Here's how the part is built. I have some questions about the finished solid (model axes, mm). A direction names the side the tool comes from. Coordinates: 2 decimals unless noted, no trailing zeros. Write each loop counter-clockwise with the first axis right and the second up, starting at its lowest first coordinate (ties: lowest second). Pieces come first, ordered by that corner, then holes. Notation, with made-up numbers: (-14.5, 4) -> (43.5, 4) arc R6 cw to (43.5, 13) -> close; hole circle Ø6 at (67, 9). An arc over 180 degrees is marked (long way). Use a Markdown table: item, result. Add a question column.
Item 1: Imagine slicing it at D-D, the plane x = 14. Write out the boundary of the cut face in (y, z).
Item 2: Will these pins go through, and if not, where does the flat tip stop? pin 1 Ø1.1 at (x, y) = (30, 19) entering from +Z; pin 2 Ø2.5 at (x, z) = (-2.125, -7) entering from -Y; pin 3 Ø0.7 at (x, y) = (-4, 18.5) entering from +Z.
Item 3: Imagine slicing it at A-A, the plane x = 4.5. Write out the boundary of the cut face in (y, z), and give its area (3 significant figures).
Item 4: If I drill on line 1 along X through (y, z) = (18.6, -7) (3 decimals); line 2 along Y through (x, z) = (19.5, -4.5); line 3 along X through (y, z) = (20.5, -1), over which ranges is the centre line in solid material (lowest first)? Write a range as from..to.
Item 5: Imagine slicing it at B-B, the plane z = -5. Write out the boundary of the cut face in (x, y).
Item 6: If we mould it in two halves opening along Z, with no side actions, what happens to faces 5 (the cylindrical face through (20.666, 28.723, -8.817)), 6 (the flat face through (-0.7, 19.2, -7.1)), 7 (the cylindrical face through (-1.126, 18.46, -6.965)), 8 (the flat face through (13, 12, 0))? For each: pulls with the +Z half, pulls with the -Z half, needs draft (parallel to the pull), parting line crosses it, or undercut.
Item 7: Imagine slicing it at C-C, the plane y = 7.5. Write out the boundary of the cut face in (x, z), and give its area (3 significant figures).
Item 8: On a 3-axis mill with a long thin cutter (end or side, diameter ignored), from which of +Z, -Z, +X, -X, +Y, -Y can I reach the whole of each face in a straight line? I mean faces 1 (the flat face through (26, 21, -7)), 2 (the flat face through (-0.7, 17.7, -7.1)), 3 (the flat face through (26.7, 17.7, -7.1)), 4 (the flat face through (16, 26.8, -7)). Say none if no direction works.
```python
from build123d import *

# Parameters (mm, degrees)
SKETCH1_W           = 26
SKETCH1_H           = 14
BOSS_EXTRUDE1_DEPTH = 22.7
SKETCH2_W           = 34.5
SKETCH2_H           = 14
BOSS_EXTRUDE2_DEPTH = 1.5
CHAMFER1_SIZE       = 1
SKETCH3_R           = 7
BOSS_EXTRUDE3_DEPTH = 26.8
SKETCH4_R           = 2.465
BOSS_EXTRUDE4_DEPTH = 3.9
SKETCH5_R           = 1
CUT_EXTRUDE1_DEPTH  = 39.466901357
SKETCH7_W           = 4.817382001
SKETCH7_H           = 1.25
SKETCH7_W_2         = 10.544713936
CUT_EXTRUDE2_DEPTH  = 39.466901357


with BuildPart() as part:
    # Sketch1 → Boss-Extrude1 (new body)
    with BuildSketch(Plane(origin=(0, 0, 0), x_dir=(1, 0, 0), z_dir=(0, 1, 0))):
        with Locations((13, 7)):
            Rectangle(SKETCH1_W, SKETCH1_H)
    extrude(amount=BOSS_EXTRUDE1_DEPTH)

    # Sketch2 → Boss-Extrude2 (add)
    with BuildSketch(Plane(origin=(0, 19.2, 0), x_dir=(1, 0, 0), z_dir=(0, 1, 0))):
        with Locations((13, 7)):
            Rectangle(SKETCH2_W, SKETCH2_H)
    extrude(amount=-BOSS_EXTRUDE2_DEPTH)

    # Chamfer1
    chamfer1_edges = [part.edges().sort_by_distance(p)[0] for p in [
        (-4.25, 18.45, -14),
        (30.25, 18.45, 0),
        (-4.25, 18.45, 0),
        (30.25, 18.45, -14),
    ]]
    chamfer(chamfer1_edges, length=CHAMFER1_SIZE)

    # Sketch3 → Boss-Extrude3 (add)
    with BuildSketch(Plane.XZ):
        with Locations(Location((19, -7, 0), (0, 0, 270))):
            Circle(SKETCH3_R)
    extrude(amount=-BOSS_EXTRUDE3_DEPTH)

    # Sketch4 → Boss-Extrude4 (add)
    with BuildSketch(Plane(origin=(0, 26.8, 0), x_dir=(1, 0, 0), z_dir=(0, 1, 0))):
        with Locations(Location((19, 7, 0), (0, 0, 270))):
            Circle(SKETCH4_R)
    extrude(amount=BOSS_EXTRUDE4_DEPTH)

    # Sketch5 → Cut-Extrude1 (cut, through all)
    with BuildSketch(Plane(origin=(0, 19.2, 0), x_dir=(1, 0, 0), z_dir=(0, 1, 0))):
        with Locations(Location((28.125, 7, 0), (0, 0, 270))):
            Circle(SKETCH5_R)
        with Locations(Location((-2.125, 7, 0), (0, 0, 270))):
            Circle(SKETCH5_R)
    extrude(amount=-CUT_EXTRUDE1_DEPTH, mode=Mode.SUBTRACT)

    # Sketch7 → Cut-Extrude2 (cut, through all)
    with BuildSketch(Plane(origin=(0, 19.2, 0), x_dir=(1, 0, 0), z_dir=(0, 1, 0))):
        with Locations((30.431785983, 7)):
            Rectangle(SKETCH7_W, SKETCH7_H)
        with Locations((-7.29545195, 7)):
            Rectangle(SKETCH7_W_2, SKETCH7_H)
    extrude(amount=-CUT_EXTRUDE2_DEPTH, mode=Mode.SUBTRACT)


solid = part.part
```
Ans:
| question | item | result |
|---|---|---|
| 1 | outline | (0, -14) -> (22.7, -14) -> (22.7, -11.9) -> (26.8, -11.9) -> (26.8, -2.1) -> (22.7, -2.1) -> (22.7, 0) -> (0, 0) -> close |
| 2 | pin 1 | stops at z = -0.2 |
| 2 | pin 2 | stops at y = 17.7 |
| 2 | pin 3 | stops at z = -0.4 |
| 3 | outline | (0, -14) -> (22.7, -14) -> (22.7, 0) -> (0, 0) -> close |
| 3 | area | 318 mm^2 |
| 4 | line 1 | x = -1.125..27.125 |
| 4 | line 2 | y = 0..26.8 |
| 4 | line 3 | x = 0..26 |
| 5 | outline | (-4.25, 17.7) -> (0, 17.7) -> (0, 0) -> (26, 0) -> (26, 17.7) -> (30.25, 17.7) -> (30.25, 19.2) -> (26, 19.2) -> (26, 22.7) -> (25.71, 22.7) -> (25.71, 26.8) -> (20.44, 26.8) -> (20.44, 30.7) -> (17.56, 30.7) -> (17.56, 26.8) -> (12.29, 26.8) -> (12.29, 22.7) -> (0, 22.7) -> (0, 19.2) -> (-4.25, 19.2) -> close |
| 6 | face 5 | parting line crosses it |
| 6 | face 6 | needs draft |
| 6 | face 7 | undercut |
| 6 | face 8 | pulls with the +Z half |
| 7 | outline | (0, -14) -> (26, -14) -> (26, 0) -> (0, 0) -> close |
| 7 | area | 364 mm^2 |
| 8 | face 1 | +Z, -Z, +X, +Y |
| 8 | face 2 | +Z, -Z, -X, -Y |
| 8 | face 3 | +Z, -Z, +X, -Y |
| 8 | face 4 | +Y |
